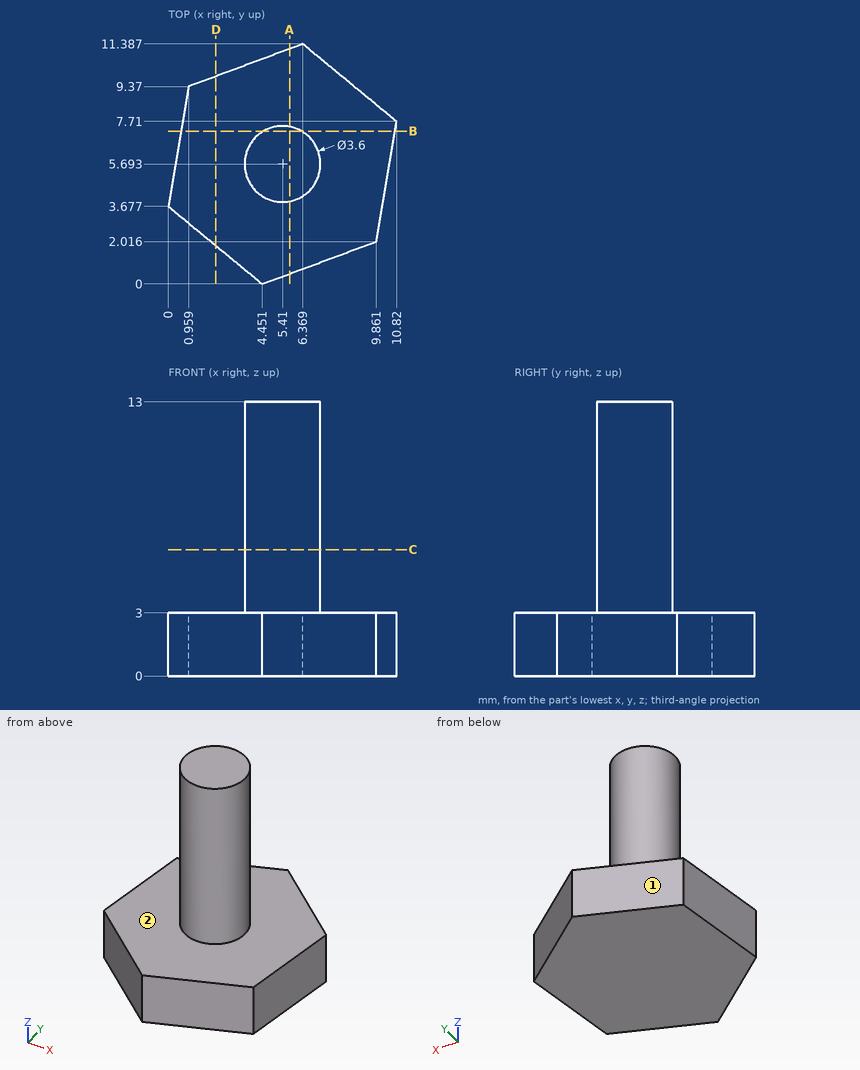
Job drawing, mm, ordinate dimensions from the low corner. One solid piece. A direction names the side the tool comes from. Round coordinates to 2 decimals unless told otherwise and drop trailing zeros. Write each loop counter-clockwise with the first axis right and the second up, starting at its lowest first coordinate (ties: lowest second). Pieces come first, ordered by that corner, then holes. Notation, with made-up numbers: M 39,-20 L 46,-20 A25 ccw 46,-4 Z; hole C 76,43.5 d3. An arc over 180 degrees is marked long. Return JSON: item names as keys, results as strings. Group by question number.
(1) Saw through at A-A on x = 5.75. Write the cut outline in (y, z) (1 decimal).
(2) Pin check, flat tips, straight feed: pin 1 Ø1.5 at (y, z) = (6, 11) entering from -X; pin 2 Ø5 at (y, z) = (2.5, 7.5) entering from -X. Stop position of each tip, or through.
(3) Which spindle directions (+Z, -Z, +X, -X, +Y, -Y) get a long thin tool onto all of the face, cutting with end or side? Do the marked faces 1 and 2. Say none if no direction does.
(4) Saw through at D-D on x = 2.25. Write the cut outline in (y, z).
(5) Saw through at C-C on z = 6. Write the cut outline in (x, y).
(6) Drill centre lines: probe 1 along Z at (x, y) = (3, 1.75); probe 2 along Y at (x, z) = (6.25, 10.75) (1 decimal); probe 3 along X at (y, z) = (8, 2.5). Where is each one in solid material? Low to high.
(7) Saw through at B-B on y = 7.25. Write the cut outline in (x, z), then the cut area to 3 significant figures.
Returned:
{
 "1": {"outline": "M 0.5,0 L 11.2,0 L 11.2,3 L 7.5,3 L 7.5,13 L 3.9,13 L 3.9,3 L 0.5,3 Z"},
 "2": {"pin 1": "x = 3.61", "pin 2": "x = 3.75"},
 "3": {"face 1": "+Z, -Z, -X, +Y", "face 2": "+Z"},
 "4": {"outline": "M 1.82,0 L 9.85,0 L 9.85,3 L 1.82,3 Z"},
 "5": {"outline": "C 5.41,5.69 d3.6"},
 "6": {"probe 1": "0 to 3", "probe 2": "4.1 to 7.3", "probe 3": "0.73 to 10.47"},
 "7": {"outline": "M 0.6,0 L 10.74,0 L 10.74,3 L 6.31,3 L 6.31,13 L 4.51,13 L 4.51,3 L 0.6,3 Z", "area": "48.5 mm²"}
}
